Geometry check sheet. Reference: drawing and pictorial views, mm from the part's lowest x, y, z. Round coordinates to 2 decimals unless told otherwise and drop trailing zeros. Order: outer loops, then holes, each group sorted by start corner. A loop starts at its lowest first (then second) coordinate and runs counter-clockwise, first axis right, second up.
(1) Sectioned sample at A-A (y = 72). Record the boundary of the cut face in (x, z), plus the area to 3 significant figures.
(2) Go/stop test with flat-tipped pins: pin 1 (1.5 mm diameter, centred on x = 84.5, z = 1.5, fed in from -Y) (1 decimal); pin 2 (8 mm diameter, centred on x = 18.74, y = 41.25, fed in from -Z); pin 3 (12 mm diameter, centred on x = 129.5, y = 75.5, fed in from -Z) (3 decimals). Record where each tip stops, or that it passes through.
(3) Material ranges on line 1 along Y through (x, z) = (72, 1.5); line 2 along X through (y, z) = (56, 0.8) (1 decimal); line 3 along X through (y, z) = (39, 1.15) (1 decimal), recorded low to high.
(4) Sectioned sample at C-C (x = 72). Record the boundary of the cut face in (y, z), plus the area to 3 significant figures.
(5) Sectioned sample at D-D (x = 10). Record the boundary of the cut face in (y, z).
(6) Sectioned sample at B-B (z = 0.6). Record the boundary of the cut face in (x, y).
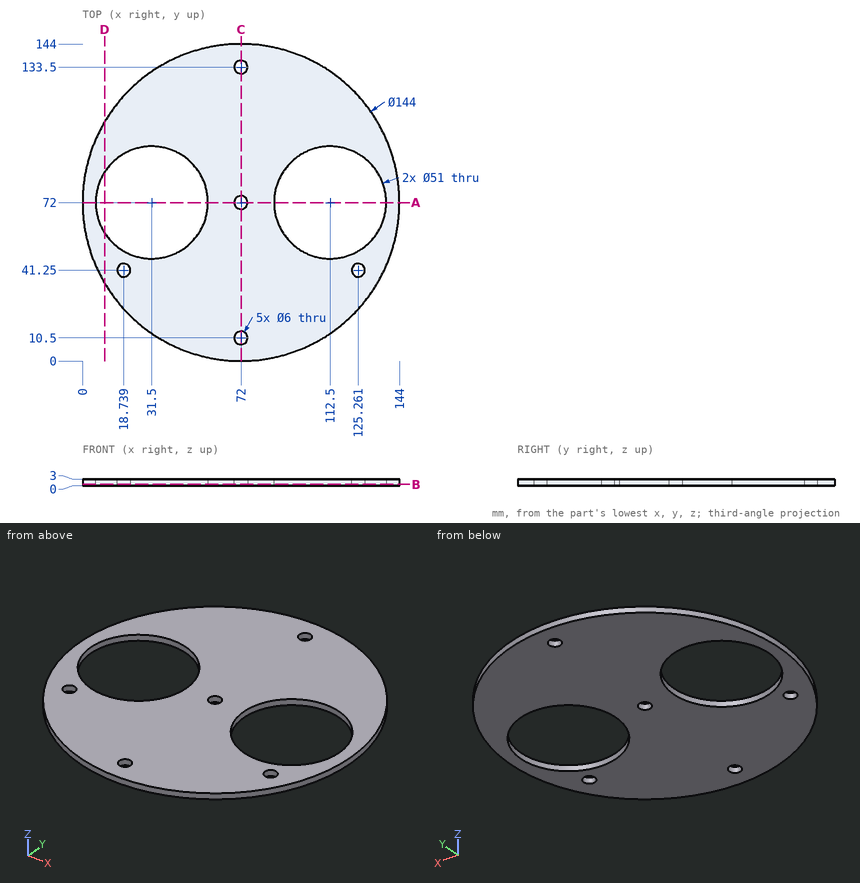
Answer below:
1. outline: (0, 0) - (6, 0) - (6, 3) - (0, 3) - close; (57, 0) - (69, 0) - (69, 3) - (57, 3) - close; (75, 0) - (87, 0) - (87, 3) - (75, 3) - close; (138, 0) - (144, 0) - (144, 3) - (138, 3) - close
1. area: 108 mm2
2. pin 1: stops at y = 1
2. pin 2: stops at z = 0
2. pin 3: passes through
3. line 1: y = 0 to 7.5, 13.5 to 69, 75 to 130.5, 136.5 to 144
3. line 2: x = 1.8 to 11.6, 51.4 to 92.6, 132.4 to 142.2
3. line 3: x = 8 to 16.8, 20.7 to 123.3, 127.2 to 136
4. outline: (0, 0) - (7.5, 0) - (7.5, 3) - (0, 3) - close; (13.5, 0) - (69, 0) - (69, 3) - (13.5, 3) - close; (75, 0) - (130.5, 0) - (130.5, 3) - (75, 3) - close; (136.5, 0) - (144, 0) - (144, 3) - (136.5, 3) - close
4. area: 378 mm2
5. outline: (35.39, 0) - (58.29, 0) - (58.29, 3) - (35.39, 3) - close; (85.71, 0) - (108.61, 0) - (108.61, 3) - (85.71, 3) - close
6. outline: circle Ø144 at (72, 72); hole circle Ø51 at (31.5, 72); hole circle Ø6 at (18.74, 41.25); hole circle Ø6 at (72, 10.5); hole circle Ø6 at (72, 72); hole circle Ø6 at (72, 133.5); hole circle Ø51 at (112.5, 72); hole circle Ø6 at (125.26, 41.25)
